Geometry: see drawing. Coordinates: mm, zero at the bounding-box minimum. Coordinates: 2 decimals unless noted, no trailing zeros. Loops run counter-clockwise (first coordinate to the right, second up) from the corner with the lowest first, then second, coordinate; pieces in that order, holes last.
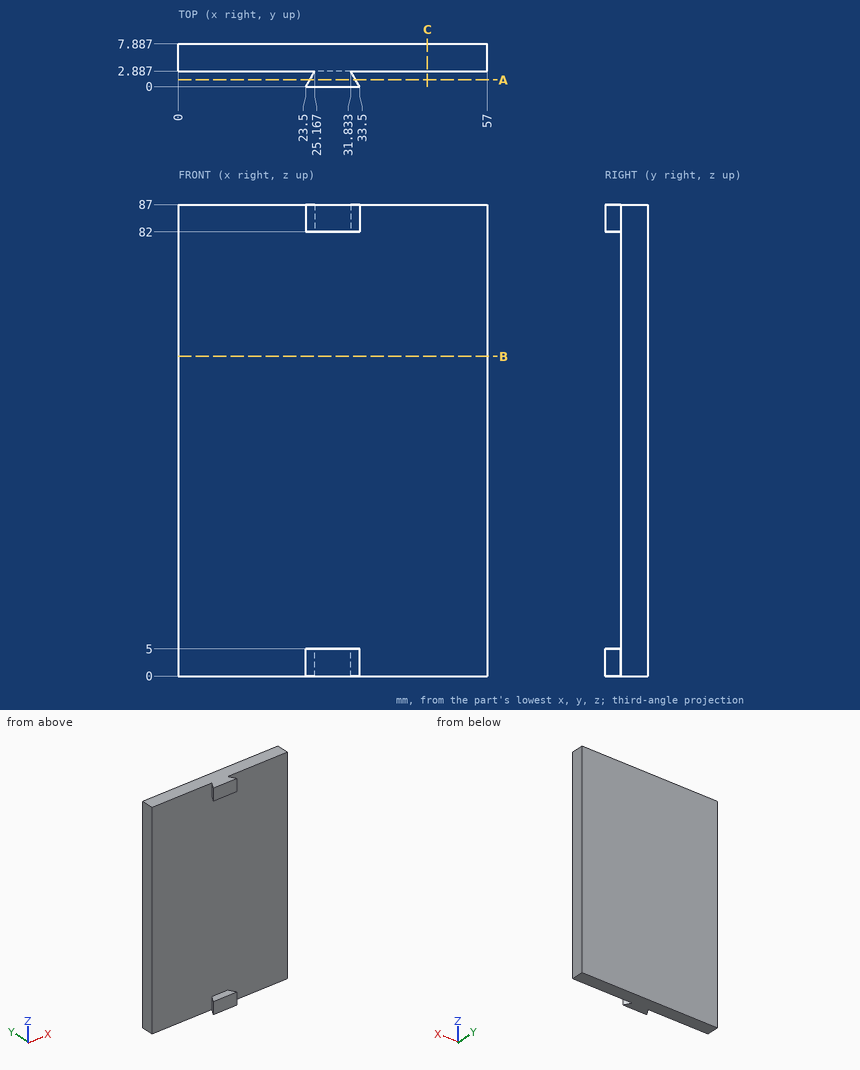
Item 1: Section query A-A (y = 1.25). Output: boundary loops of the cut face in (x, z).
Result:
outline: (24.22, 0) - (32.78, 0) - (32.78, 5) - (24.22, 5) - close; (24.22, 82) - (32.78, 82) - (32.78, 87) - (24.22, 87) - close
Item 2: Contact query for a flat-ended pin moving along its axis: P1, Ø5, axis at x = 7.5, z = 14.5, coming from the -Y side. Output: stop coordinate, or through.
Result:
P1: stops at y = 2.89
Item 3: Line query: L1, parallel to Y at x = 15.5, z = 67. Output: solid intervals per line, ascending.
Result:
L1: y = 2.89 to 7.89
Item 4: Section query B-B (z = 59). Output: boundary loops of the cut face in (x, y).
Result:
outline: (0, 2.89) - (57, 2.89) - (57, 7.89) - (0, 7.89) - close
Item 5: Section query C-C (x = 46). Output: boundary loops of the cut face in (y, z).
Result:
outline: (2.89, 0) - (7.89, 0) - (7.89, 87) - (2.89, 87) - close
